```python
from build123d import *

# Parameters (mm, degrees)
SKETCH1_W           = 5.842
SKETCH1_H           = 12.7
BOSS_EXTRUDE1_DEPTH = 5.842
SKETCH2_R           = 0.1984375
CUT_EXTRUDE1_DEPTH  = 5.842


with BuildPart() as part:
    # Sketch1 → Boss-Extrude1 (new body)
    with BuildSketch(Plane.XY):
        Polygon((2.159, -25.4), (-9.017, -3.175), (-9.017, 22.225), (6.35, 22.225), (12.192, 22.225), (27.559, 22.225), (27.559, -25.4), align=None)
        with Locations((-2.921, 6.35)):
            Rectangle(SKETCH1_W, SKETCH1_H, mode=Mode.SUBTRACT)
        Polygon((12.192, 0), (12.192, -12.7), (12.192, -19.05), (6.35, -19.05), (6.35, -12.7), (6.35, 0), (6.35, 19.05), (12.192, 19.05), align=None, mode=Mode.SUBTRACT)
        with Locations((21.463, 6.35)):
            Rectangle(SKETCH1_W, SKETCH1_H, mode=Mode.SUBTRACT)
    extrude(amount=BOSS_EXTRUDE1_DEPTH)

    # Sketch2 → Cut-Extrude1 (cut)
    with BuildSketch(Plane.XY.offset(5.842)):
        with Locations((-5.842, 12.7)):
            Circle(SKETCH2_R)
        with Locations((0, 12.7)):
            Circle(SKETCH2_R)
        Circle(SKETCH2_R)
        with Locations((-5.842, 0)):
            Circle(SKETCH2_R)
        with Locations((24.384, 0)):
            Circle(SKETCH2_R)
        with Locations((18.542, 0)):
            Circle(SKETCH2_R)
        with Locations((18.542, 12.7)):
            Circle(SKETCH2_R)
        with Locations((24.384, 12.7)):
            Circle(SKETCH2_R)
    extrude(amount=-CUT_EXTRUDE1_DEPTH, mode=Mode.SUBTRACT)


solid = part.part
```
Work out the finished part from the listing and answer in its coordinate system (mm). A direction names the side the tool comes from. Round coordinates to 2 decimals unless told otherwise and drop trailing zeros. Loops run counter-clockwise (first coordinate to the right, second up) from the corner with the lowest first, then second, coordinate; pieces in that order, holes last. Notation, with made-up numbers: M 29.25,74.25 L 72.25,74.25 A32 cw 72.25,110.25 Z; hole C 39,71 d9. An arc over 180 degrees is marked long. One line per question, with ' | ' between items.
Q1. Find section A-A, the plane x = 21. Give the vertices of the cut face in (y, z) (3 decimals).
Conclusion:
outline: M -25.4,0 L 0,0 L 0,5.842 L -25.4,5.842 Z; M 12.7,0 L 22.225,0 L 22.225,5.842 L 12.7,5.842 Z
Q2. Find section D-D, the plane x = 1. Give the vertices of the cut face in (y, z) (3 decimals).
Conclusion:
outline: M -23.095,0 L 22.225,0 L 22.225,5.842 L -23.095,5.842 Z
Q3. Find section B-B, the plane y = 2.5. Give the vertices of the cut face in (x, z).
Conclusion:
outline: M -9.02,0 L -5.84,0 L -5.84,5.84 L -9.02,5.84 Z; M 0,0 L 6.35,0 L 6.35,5.84 L 0,5.84 Z; M 12.19,0 L 18.54,0 L 18.54,5.84 L 12.19,5.84 Z; M 24.38,0 L 27.56,0 L 27.56,5.84 L 24.38,5.84 Z
Q4. Find section C-C, the plane z = 3.7. Give the vertices of the cut face in (x, y) (3 decimals), then the cut area to 3 significant figures.
Conclusion:
outline: M -9.017,-3.175 L 2.159,-25.4 L 27.559,-25.4 L 27.559,22.225 L -9.017,22.225 Z; hole M -5.842,0.198 A0.198 ccw long -5.644,0 L -0.198,0 A0.198 ccw long 0,0.198 L 0,12.502 A0.198 ccw long -0.198,12.7 L -5.644,12.7 A0.198 ccw long -5.842,12.502 Z; hole M 6.35,-19.05 L 12.192,-19.05 L 12.192,19.05 L 6.35,19.05 Z; hole M 18.542,0.198 A0.198 ccw long 18.74,0 L 24.186,0 A0.198 ccw long 24.384,0.198 L 24.384,12.502 A0.198 ccw long 24.186,12.7 L 18.74,12.7 A0.198 ccw long 18.542,12.502 Z | area: 1,250 mm2
Q5. A tool of negligible diameter and unlimited length cuts with its end or side. For faces 1 (the flat face through (9, -19.05, 3)), 2 (the flat face through (14, -1, 0)), from which of +Z, -Z, +X, -X, +Y, -Y can it reach the whole face along a straight path? Write none if from no direction.
Conclusion:
face 1: +Z, -Z | face 2: -Z, +X, -X, +Y, -Y
Q6. Consider line 1 along X through (y, z) = (1, 1.4); line 2 along Y through (x, z) = (22, 1.6) (3 decimals); line 3 along Y through (x, z) = (9, 1.1) (3 decimals). Determine where each line is inside the solid, lowest interval first. Write a range as from..to.
Conclusion:
line 1: x = -9.02..-5.84, 0..6.35, 12.19..18.54, 24.38..27.56 | line 2: y = -25.4..0, 12.7..22.225 | line 3: y = -25.4..-19.05, 19.05..22.225
Q7. Each of these flat-tipped pins is pushed along its axis until it touches: pin 1 Ø1.5 at (x, z) = (-2, 4.5) entering from -Y; pin 2 Ø10 at (x, y) = (8, -3) entering from +Z. Where does it stop, or does it pass through?
Conclusion:
pin 1: stops at y = -18.62 | pin 2: stops at z = 5.84
Q8. The mould has two halves that part along X. Classify faces 3 (the flat face through (-3, 0, 3)), 4 (the flat face through (14, -1, 5.842)), 5 (the flat face through (27.559, -1, 3)): +X half, -X half, draft (parallel to the pull), parting line (faces both ways), or undercut.
Conclusion:
face 3: undercut | face 4: draft | face 5: +X half
